Can you work these out from the drawing? Everything is in mm from the part's minimum corner. Give positions to 0.01 mm unless a question says otherwise; leave off trailing zeros. Write each loop counter-clockwise with the first axis right and the second up, starting at its lowest first coordinate (ties: lowest second). Pieces come first, ordered by that corner, then holes. Notation, with made-up numbers: (82.5, -25) - (92.5, -25) arc R12 ccw to (92.5, -11) - close; hole circle Ø1 at (-30.75, 18.5). An arc over 180 degrees is marked (long way). Write each question's results on one line, items separated by ' | '. Start each with the question number.
Item 1: Suppose I cut it at A-A on y = 2.3. List the corners of the cut face in (x, z) for me (1 decimal), then the cut area to 3 significant figures.
Item 2: Suppose I cut it at B-B on x = 92. List the corners of the cut face in (y, z) for me, then the cut area to 3 significant figures.
Item 3: Please list where these lines run through material, in increasing order: line 1 along Z through (x, y) = (185, 1); line 2 along X through (y, z) = (1.8, 10); line 3 along X through (y, z) = (3.7, 11).
Item 4: Will these pins go through, and if not, where does the flat tip stop? P1, Ø1.8, axis at x = 35, z = 10, coming from the -Y side; P2, Ø2, axis at y = 3.5, z = 7.5, coming from the +X side.
Item 5: Suppose I cut it at C-C on z = 14. List the corners of the cut face in (x, y) for me, then the cut area to 3 significant figures.
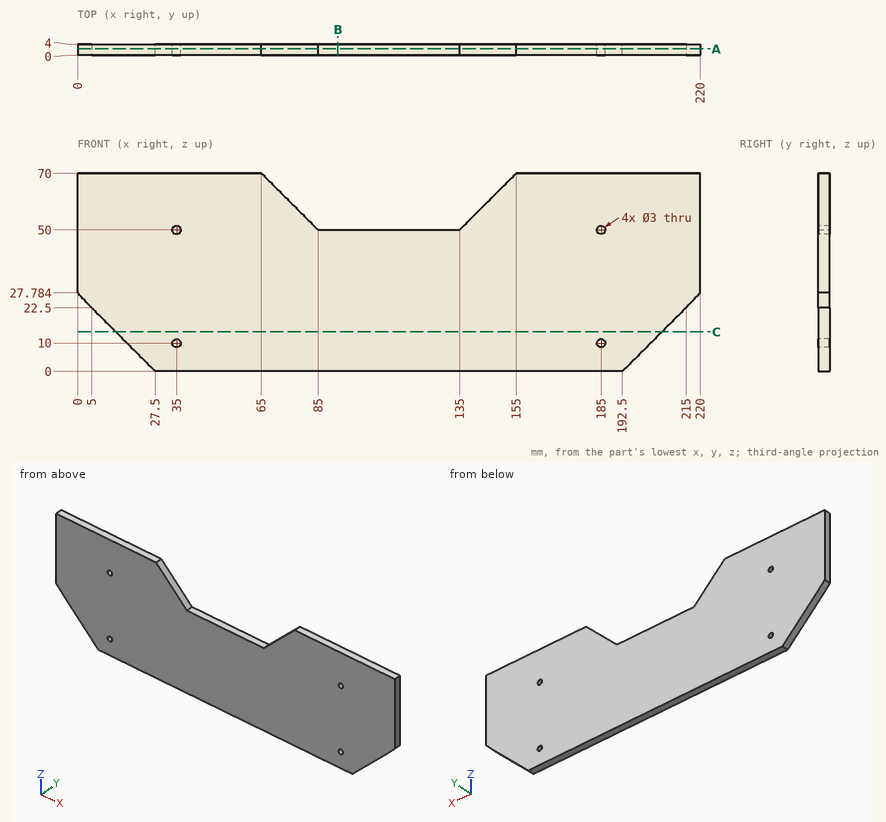
Checked values:
1) outline: (0, 27.8) - (5, 22.5) - (27.5, 0) - (192.5, 0) - (215, 22.5) - (220, 27.8) - (220, 70) - (155, 70) - (135, 50) - (85, 50) - (65, 70) - (0, 70) - close; hole circle Ø3 at (35, 10); hole circle Ø3 at (35, 50); hole circle Ø3 at (185, 10); hole circle Ø3 at (185, 50) | area: 13,200 mm^2
2) outline: (0, 0) - (4, 0) - (4, 50) - (0, 50) - close | area: 200 mm^2
3) line 1: z = 0 to 8.5, 11.5 to 48.5, 51.5 to 70 | line 2: x = 17.5 to 33.5, 36.5 to 183.5, 186.5 to 202.5 | line 3: x = 16.5 to 33.88, 36.12 to 183.88, 186.12 to 203.5
4) P1: passes through | P2: stops at x = 201
5) outline: (13.5, 0) - (206.5, 0) - (206.5, 4) - (13.5, 4) - close | area: 772 mm^2
